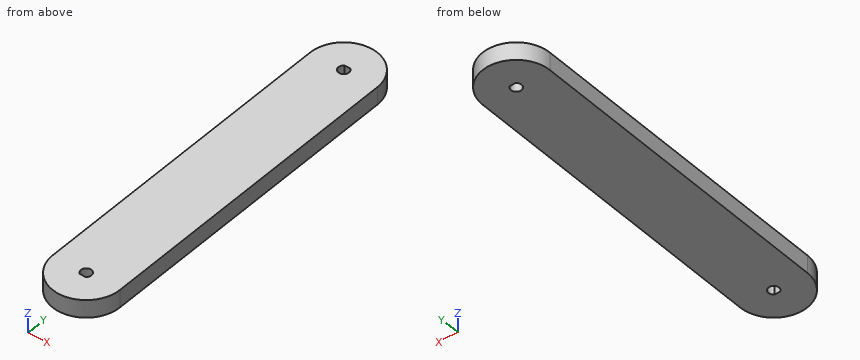
```python
from build123d import *

# Parameters (mm, degrees)
EXTRUDE_1_DEPTH = 10


with BuildPart() as part:
    # 草图1 → 凸台-拉伸1 (new body)
    with BuildSketch(Plane.XY):
        with BuildLine():
            Line((19, -90), (19, 90))
            ThreePointArc((19, 90), (0, 109), (-19, 90))
            Line((-19, 90), (-19, -90))
            ThreePointArc((-19, -90), (0, -109), (19, -90))
        make_face()
        with BuildLine():
            ThreePointArc((-1.658312395, -92.5), (0, -87), (1.658312395, -92.5))
            Line((1.658312395, -92.5), (-1.658312395, -92.5))
        make_face(mode=Mode.SUBTRACT)
        with BuildLine():
            Line((-1.658312395, 92.5), (1.658312395, 92.5))
            ThreePointArc((1.658312395, 92.5), (0, 87), (-1.658312395, 92.5))
        make_face(mode=Mode.SUBTRACT)
    extrude(amount=EXTRUDE_1_DEPTH)


solid = part.part
```
CAD build for the part. Positions are in the model's coordinates, mm. Coordinates: 2 decimals unless noted, no trailing zeros. Order: outer loops, then holes, each group sorted by start corner. A loop starts at its lowest first (then second) coordinate and runs counter-clockwise, first axis right, second up. Notation, with made-up numbers: (4, 69) - (55, 69) arc R19 cw to (55, 91) - close; hole circle Ø9 at (-1.5, 56). An arc over 180 degrees is marked (long way). Use a Markdown table: item, result. Add a question column.
(1) Drill centre lines: line 1 along Y through (x, z) = (0, 7); line 2 along Y through (x, z) = (-2, 8.5); line 3 along X through (y, z) = (90, 7). Where is each one in solid material? Low to high. Write a range as [from, to].
(2) Flat gauge pins, fed straight in: pin 1 (5 mm diameter, centred on x = -5, z = 3, fed in from +Y); pin 2 (3.5 mm diameter, centred on x = 1, z = 2.5, fed in from -Y); pin 3 (1 mm diameter, centred on x = 0, z = 6, fed in from +Y). Where does each tip first touch, or does it go through?
(3) Saw through at A-A (z = 6.5). Give the cut face in (x, y).
(4) Saw through at B-B (y = -95). Give the cut face in (x, z).
(5) Saw through at C-C (x = -11.5). Give the cut face in (y, z), then the cut area to 3 significant figures.
Solved:
| question | item | result |
|---|---|---|
| 1 | line 1 | y = [-109, -92.5], [-87, 87], [92.5, 109] |
| 1 | line 2 | y = [-108.89, -92.24], [-87.76, 87.76], [92.24, 108.89] |
| 1 | line 3 | x = [-19, -3], [3, 19] |
| 2 | pin 1 | stops at y = 108.83 |
| 2 | pin 2 | stops at y = -109 |
| 2 | pin 3 | stops at y = 109 |
| 3 | outline | (-19, -90) arc R19 ccw to (19, -90) - (19, 90) arc R19 ccw to (-19, 90) - close; hole (-1.66, -92.5) - (1.66, -92.5) arc R3 ccw (long way) to start; hole (-1.66, 92.5) arc R3 ccw (long way) to (1.66, 92.5) - close |
| 4 | outline | (-18.33, 0) - (18.33, 0) - (18.33, 10) - (-18.33, 10) - close |
| 5 | outline | (-105.12, 0) - (105.12, 0) - (105.12, 10) - (-105.12, 10) - close |
| 5 | area | 2,100 mm² |
